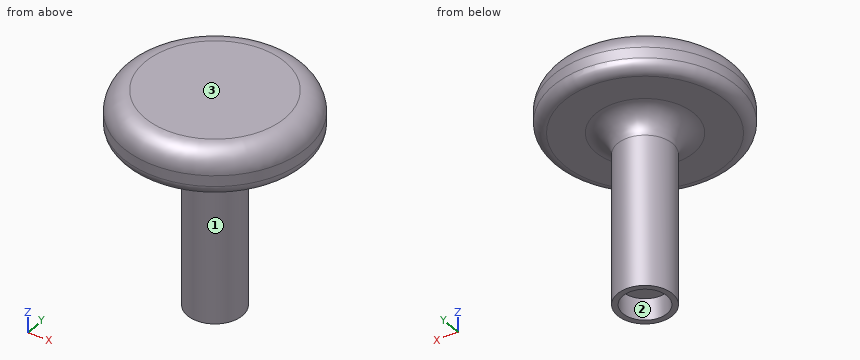
```python
from build123d import *

# Parameters (mm, degrees)
CROQUIS1_R              = 12.75
SALIENTE_EXTRUIR1_DEPTH = 80
CROQUIS2_R              = 42.5
SALIENTE_EXTRUIR2_DEPTH = 20
REDONDEO1_R             = 10
CROQUIS3_R              = 10.25
CORTAR_EXTRUIR1_DEPTH   = 10
REDONDEO2_R             = 10
REDONDEO3_R             = 5


with BuildPart() as part:
    # Croquis1 → Saliente-Extruir1 (new body)
    with BuildSketch(Plane.XY):
        Circle(CROQUIS1_R)
    extrude(amount=SALIENTE_EXTRUIR1_DEPTH)

    # Croquis2 → Saliente-Extruir2 (add)
    with BuildSketch(Plane.XY.offset(80)):
        Circle(CROQUIS2_R)
    extrude(amount=SALIENTE_EXTRUIR2_DEPTH)

    # Redondeo1
    redondeo1_edges = [part.edges().sort_by_distance(p)[0] for p in [
        (-42.5, 0, 100),
    ]]
    fillet(redondeo1_edges, radius=REDONDEO1_R)

    # Croquis3 → Cortar-Extruir1 (cut)
    with BuildSketch(Plane(origin=(0, 0, 0), x_dir=(-1, 0, 0), z_dir=(0, 0, -1))):
        Circle(CROQUIS3_R)
    extrude(amount=-CORTAR_EXTRUIR1_DEPTH, mode=Mode.SUBTRACT)

    # Redondeo2
    redondeo2_edges = [part.edges().sort_by_distance(p)[0] for p in [
        (-12.75, 0, 80),
    ]]
    fillet(redondeo2_edges, radius=REDONDEO2_R)

    # Redondeo3
    redondeo3_edges = [part.edges().sort_by_distance(p)[0] for p in [
        (-42.5, 0, 80),
    ]]
    fillet(redondeo3_edges, radius=REDONDEO3_R)


solid = part.part
```
Here's how the part is built. I have some questions about the finished solid (model axes, mm). Face numbers are marked on the shaded views. Coordinates: 2 decimals unless noted, no trailing zeros. Loops run counter-clockwise (first coordinate to the right, second up) from the corner with the lowest first, then second, coordinate; pieces in that order, holes last. Notation, with made-up numbers: M 25.5,-10 L 65.5,-10 A16 cw 65.5,5 Z; hole C 33,15 d11. An arc over 180 degrees is marked long. One line per item, written item: value.
1. Will these pins go through, and if not, where does the flat tip stop? pin 1 Ø8 at (x, z) = (-6, 50.5) entering from -Y; pin 2 Ø8 at (y, z) = (-4.5, 70.5) entering from +X; pin 3 Ø1 at (x, z) = (10.5, 67.5) entering from +Y.
Geometry says:
pin 1: stops at y = -12.59
pin 2: stops at x = 13.35
pin 3: stops at y = 7.91
2. Imagine slicing it at A-A (x = 0). List the corners of the cut face in (y, z) for me.
Geometry says:
outline: M -42.5,85 A5 ccw -37.5,80 L -22.75,80 A10 cw -12.75,70 L -12.75,0 L -10.25,0 L -10.25,10 L 10.25,10 L 10.25,0 L 12.75,0 L 12.75,70 A10 cw 22.75,80 L 37.5,80 A5 ccw 42.5,85 L 42.5,90 A10 ccw 32.5,100 L -32.5,100 A10 ccw -42.5,90 Z
3. Please list where these lines run through material, in increasing order: probe 1 along Y at (x, z) = (0, 2); probe 2 along Z at (x, y) = (-6.5, 29.5); probe 3 along X at (y, z) = (0.5, 20).
Geometry says:
probe 1: y = -12.75 to -10.25, 10.25 to 12.75
probe 2: z = 80 to 100
probe 3: x = -12.74 to 12.74
4. Imagine slicing it at C-C (z = 34). List the corners of the cut face in (x, y) for me, and give its area (3 significant figures).
Geometry says:
outline: C 0,0 d25.5
area: 511 mm2
5. Thinking about a two-plate mould opening in Y: for the marked faces 1, 2 and 3, which applies, +Y half, -Y half, draft (parallel to the pull), parting line (faces both ways), or undercut?
Geometry says:
face 1: parting line
face 2: undercut
face 3: draft
